Part model, mm, in its own coordinate system. A direction names the side the tool comes from. Give positions to 0.01 mm unless a question says otherwise; leave off trailing zeros. Order: outer loops, then holes, each group sorted by start corner. A loop starts at its lowest first (then second) coordinate and runs counter-clockwise, first axis right, second up. Notation, with made-up numbers: M 62,-20.5 L 75,-20.5 A32 ccw 75,6.5 Z; hole C 16.5,61.5 d1. An arc over 180 degrees is marked long. Return JSON: item names as keys, results as strings.
from build123d import *

# Parameters (mm, degrees)
SKETCH1_R           = 11
BOSS_EXTRUDE1_DEPTH = 6.5
SKETCH2_R           = 9
BOSS_EXTRUDE2_DEPTH = 5.5
SKETCH3_R           = 3
CUT_EXTRUDE1_DEPTH  = 13
SKETCH4_R           = 1.5
BOSS_EXTRUDE3_DEPTH = 3.5
CIRPATTERN1_COUNT   = 3
SKETCH5_R           = 10.95
SKETCH5_R_2         = 3.1
BOSS_EXTRUDE4_DEPTH = 3
SKETCH7_R           = 2
CUT_EXTRUDE2_DEPTH  = 12


with BuildPart() as part:
    # Sketch1 → Boss-Extrude1 (new body)
    with BuildSketch(Plane(origin=(0, 0, 0), x_dir=(1, 0, 0), z_dir=(0, 1, 0))):
        Circle(SKETCH1_R)
    extrude(amount=BOSS_EXTRUDE1_DEPTH)

    # Sketch2 → Boss-Extrude2 (add)
    with BuildSketch(Plane(origin=(0, 6.5, 0), x_dir=(1, 0, 0), z_dir=(0, 1, 0))):
        Circle(SKETCH2_R)
    extrude(amount=BOSS_EXTRUDE2_DEPTH)

    # Sketch3 → Cut-Extrude1 (cut, through all)
    with BuildSketch(Plane(origin=(0, 12, 0), x_dir=(1, 0, 0), z_dir=(0, 1, 0))):
        Circle(SKETCH3_R)
    extrude(amount=-CUT_EXTRUDE1_DEPTH, mode=Mode.SUBTRACT)

    # Sketch4 → Boss-Extrude3 (add)
    with BuildSketch(Plane(origin=(0, 12, 0), x_dir=(1, 0, 0), z_dir=(0, 1, 0))):
        with Locations((0, 6.2)):
            Circle(SKETCH4_R)
    boss_extrude3 = extrude(amount=BOSS_EXTRUDE3_DEPTH)

    # CirPattern1: Boss-Extrude3 ×3 about axis
    cirpattern1_axis = Axis((0, 0, 0), (0, 1, 0))
    for i in range(1, CIRPATTERN1_COUNT):
        add(boss_extrude3.rotate(cirpattern1_axis, i * 360 / CIRPATTERN1_COUNT))

    # Sketch5 → Boss-Extrude4 (add)
    with BuildSketch(Plane(origin=(0, 15.5, 0), x_dir=(1, 0, 0), z_dir=(0, 1, 0))):
        Circle(SKETCH5_R)
        Circle(SKETCH5_R_2, mode=Mode.SUBTRACT)
    extrude(amount=BOSS_EXTRUDE4_DEPTH)

    # Sketch7 → Cut-Extrude2 (cut, through all)
    with BuildSketch(Plane.XY):
        with Locations((0, 3.25)):
            Circle(SKETCH7_R)
    extrude(amount=CUT_EXTRUDE2_DEPTH, mode=Mode.SUBTRACT)


solid = part.part
Q1. Probe line 1 along Y through (x, z) = (0, 4.75); line 2 along Y through (x, z) = (8, 6.25); line 3 along Z through (x, y) = (0, 9). List the from-to ranges inside material, lowest first.
Established:
{"line 1": "y = 0 to 1.25, 5.25 to 12, 15.5 to 18.5", "line 2": "y = 0 to 6.5, 15.5 to 18.5", "line 3": "z = -9 to -3, 3 to 9"}
Q2. Band-saw the part on C-C (x = -8.25). Give the cut face in (y, z), then the cut area to 3 significant figures.
Established:
{"outline": "M 0,-7.28 L 6.5,-7.28 L 6.5,-3.6 L 12,-3.6 L 12,3.6 L 6.5,3.6 L 6.5,7.28 L 0,7.28 Z; M 15.5,-7.2 L 18.5,-7.2 L 18.5,7.2 L 15.5,7.2 Z", "area": "177 mm²"}
Q3. Band-saw the part on D-D (y = 7.5). Give the cut face in (x, z).
Established:
{"outline": "C 0,0 d18; hole C 0,0 d6"}
Q4. Band-saw the part on B-B (z = 0). Give the cut face in (x, y).
Established:
{"outline": "M -11,0 L -3,0 L -3,12 L -9,12 L -9,6.5 L -11,6.5 Z; M -10.95,15.5 L -3.1,15.5 L -3.1,18.5 L -10.95,18.5 Z; M 3,0 L 11,0 L 11,6.5 L 9,6.5 L 9,12 L 3,12 Z; M 3.1,15.5 L 10.95,15.5 L 10.95,18.5 L 3.1,18.5 Z"}
Q5. Pin check, flat tips, straight feed: pin 1 (7 mm diameter, centred on x = 0, z = 0, fed in from -Y); pin 2 (5 mm diameter, centred on y = 12, z = -4.5, fed in from -X); pin 3 (2 mm diameter, centred on x = -7.5, y = 11, fed in from +Z); pin 4 (2 mm diameter, centred on x = -3.5, y = 9, fed in from +Z). Stop position of each tip, or through.
Established:
{"pin 1": "stops at y = 0", "pin 2": "stops at x = -8.77", "pin 3": "stops at z = 6.22", "pin 4": "stops at z = 8.65"}
Q6. Two-plate mould, pull along Z, no slides. Class faces 1 (the cylindrical face through (-2.38, 3.2, 10.74)), 2 (the flat face through (4, 12, 0)), 3 (the cylindrical face through (1.43, 16.98, 2.75)): +Z half, -Z half, draft (parallel to the pull), parting line (faces both ways), or undercut.
Established:
{"face 1": "parting line", "face 2": "draft", "face 3": "undercut"}
Q7. 3-axis set-ups, long thin cutter, end or side, ignore diameter. For faces 4 (the cylindrical face through (-1.172, 9.212, -8.923)), 5 (the cylindrical face through (-8.69, 16.98, 6.66)), 6 (the cylindrical face through (-2, 3.3, 6.6)): which of +Z, -Z, +X, -X, +Y, -Y reach the whole face in a straight line?
Established:
{"face 4": "none", "face 5": "+Y", "face 6": "+Z"}
Q8. Band-saw the part on A-A (x = 0). Give the cut face in (y, z), then the cut area to 3 significant figures.
Established:
{"outline": "M 0,-11 L 6.5,-11 L 6.5,-9 L 12,-9 L 12,-7.7 L 15.5,-7.7 L 15.5,-10.95 L 18.5,-10.95 L 18.5,-3.1 L 15.5,-3.1 L 15.5,-4.7 L 12,-4.7 L 12,-3 L 0,-3 Z; M 0,3 L 1.25,3 L 1.25,11 L 0,11 Z; M 5.25,3 L 12,3 L 12,9 L 6.5,9 L 6.5,11 L 5.25,11 Z; M 15.5,3.1 L 18.5,3.1 L 18.5,10.95 L 15.5,10.95 Z", "area": "196 mm²"}
